from build123d import *

# Parameters (mm, degrees)
SKETCH1_W           = 20
SKETCH1_H           = 20
BOSS_EXTRUDE1_DEPTH = 150
SKETCH2_W           = 7
SKETCH2_H           = 21
SKETCH2_W_2         = 21
SKETCH2_H_2         = 7
BOSS_EXTRUDE2_DEPTH = 2


with BuildPart() as part:
    # Sketch1 → Boss-Extrude1 (new body)
    with BuildSketch(Plane.XY):
        Polygon((22.477189953, 38), (-22.477189953, 38), (-16.268065934, 16.268065934), (-38, 22.477189953), (-38, -22.477189953), (-16.268065934, -16.268065934), (-22.477189953, -38), (22.477189953, -38), (16.268065934, -16.268065934), (38, -22.477189953), (38, 22.477189953), (16.268065934, 16.268065934), align=None)
        Polygon((12.5, 14), (-12.5, 14), (-18.5, 35), (18.5, 35), align=None, mode=Mode.SUBTRACT)
        Rectangle(SKETCH1_W, SKETCH1_H, mode=Mode.SUBTRACT)
        Polygon((14, -12.5), (14, 12.5), (35, 18.5), (35, -18.5), align=None, mode=Mode.SUBTRACT)
        Polygon((-12.5, -14), (12.5, -14), (18.5, -35), (-18.5, -35), align=None, mode=Mode.SUBTRACT)
        Polygon((-14, 12.5), (-14, -12.5), (-35, -18.5), (-35, 18.5), align=None, mode=Mode.SUBTRACT)
    extrude(amount=BOSS_EXTRUDE1_DEPTH)

    # Sketch2 → Boss-Extrude2 (add)
    with BuildSketch(Plane.XY):
        with Locations((0, 24.5)):
            Rectangle(SKETCH2_W, SKETCH2_H)
        with Locations((24.5, 0)):
            Rectangle(SKETCH2_W_2, SKETCH2_H_2)
        with Locations((0, -24.5)):
            Rectangle(SKETCH2_W, SKETCH2_H)
        with Locations((-24.5, 0)):
            Rectangle(SKETCH2_W_2, SKETCH2_H_2)
    extrude(amount=BOSS_EXTRUDE2_DEPTH)


solid = part.part
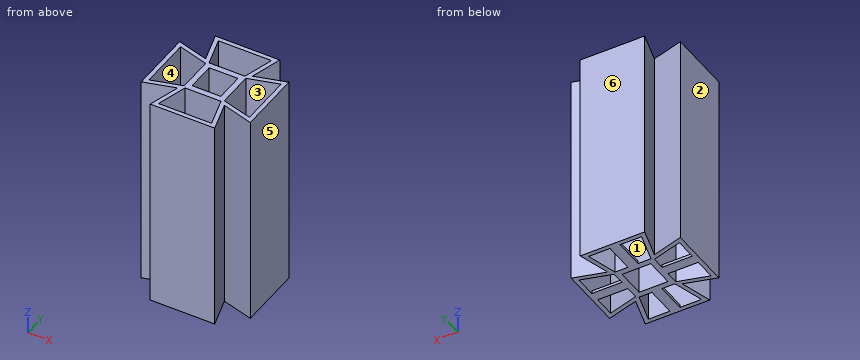
Design review of the part built by this model. Coordinates are the model's own, in mm. Face numbers are marked on the shaded views. A direction names the side the tool comes from. Coordinates: 2 decimals unless noted, no trailing zeros. Order: outer loops, then holes, each group sorted by start corner. A loop starts at its lowest first (then second) coordinate and runs counter-clockwise, first axis right, second up. Notation, with made-up numbers: (1.25, -19.75) -> (32.25, -19.75) arc R16 ccw to (32.25, 6.25) -> close; hole circle Ø11 at (87.25, 29.5). An arc over 180 degrees is marked (long way). Use one line per item in the form item = value. Start each with the question number.
(1) The part is to be moulded in two halves that separate along X. For the marked faces 4, 5 and 6, say which applies: +X half, -X half, draft (parallel to the pull), parting line (faces both ways), or undercut.
(2) Insertion check: pin 1 (7.5 mm diameter, centred on x = -0.5, y = -26, fed in from +Z); pin 2 (0.6 mm diameter, centred on x = -25.5, z = 1, fed in from -Y); pin 3 (2 mm diameter, centred on x = 25.5, z = 0.5, fed in from +Y). Each pin has a flat end and moves straight along its axis. Give the tip position at first contact, or say it passes through.
(3) For the marked faces 1, 2 and 3, list the 3-axis set-ups (+Z, -Z, +X, -X, +Y, -Y) from which the entire face can be reached by the end or side of a thin tool; tool diameter is ignored.
(4) For probe 1 along X at (y, z) = (-4.5, 144.5); probe 2 along X at (y, z) = (10.5, 71), list the stretches that pass through material, from the lowest coordinate up.
(5) Add section B-B on z = 70. Give the number of separate pieces and of enclosed holes in the cut face, plus the area to 3 significant figures.
(6) Add section A-A on y = 6.5. State the section outline as (x, z) points.
(7) Add section C-C on y = 26. State the section outline as (x, z) points, plus the area to 3 significant figures.
Answer block:
q1.face_4 = undercut
q1.face_5 = +X half
q1.face_6 = draft
q2.pin_1 = 2
q2.pin_2 = -18.99
q2.pin_3 = 19.19
q3.face_1 = +Z
q3.face_2 = +Z, -Z, -X, +Y, -Y
q3.face_3 = +Z, -Z
q4.probe_1 = -38 to -35, -14 to -10, 10 to 14, 35 to 38
q4.probe_2 = -38 to -35, -14 to 14, 35 to 38
q5.separate_pieces = 1
q5.enclosed_holes = 5
q5.area = 1,420 mm²
q6.outline = (-38, 0) -> (-35, 0) -> (-35, 150) -> (-38, 150) -> close; (-14, 0) -> (-10, 0) -> (-10, 150) -> (-14, 150) -> close; (10, 0) -> (14, 0) -> (14, 150) -> (10, 150) -> close; (35, 0) -> (38, 0) -> (38, 150) -> (35, 150) -> close
q7.outline = (-19.05, 0) -> (-15.93, 0) -> (-15.93, 150) -> (-19.05, 150) -> close; (-3.5, 0) -> (3.5, 0) -> (3.5, 2) -> (-3.5, 2) -> close; (15.93, 0) -> (19.05, 0) -> (19.05, 150) -> (15.93, 150) -> close
q7.area = 950 mm²
